Geometry: final body of the model. Coordinates: model frame, mm. Face numbers are marked on the shaded views. Coordinates: 2 decimals unless noted, no trailing zeros. Loops run counter-clockwise (first coordinate to the right, second up) from the corner with the lowest first, then second, coordinate; pieces in that order, holes last. Notation, with made-up numbers: (7.25, -11) - (53.25, -11) arc R15 cw to (53.25, 5) - close; hole circle Ø4 at (41, 60). An arc over 180 degrees is marked (long way). Put each result on its own line as item: value. Start each with the question number.
1) Material intervals for line 1 along Z through (x, y) = (0, 3.75); line 2 along Z through (x, y) = (2.5, 10.25), sorted ascending. Write a range as from..to.
2) Section A-A on z = 0. Output: boundary loops of the cut face in (x, y), and give its area (3 significant figures).
3) Section D-D on y = 13.25. Output: boundary loops of the cut face in (x, z), and give its area (3 significant figures).
4) Contact query for flat-ended pins moving along their axis: pin 1 Ø1.5 at (x, y) = (1, 3) entering from +Z; pin 2 Ø4 at (y, z) = (3.5, 0.5) entering from +X; pin 3 Ø3 at (y, z) = (11, 1) entering from -X. Output: stop coordinate, or through.
5) Draft query along X for the marked faces 1, 2, 3 and 4. Return one class per face: +X half, -X half, draft (parallel to the pull), parting line (faces both ways), or undercut.
6) Section B-B on x = 0.75. Output: boundary loops of the cut face in (y, z).
7) Section C-C on x = 3.25. Output: boundary loops of the cut face in (y, z), and give its area (3 significant figures).
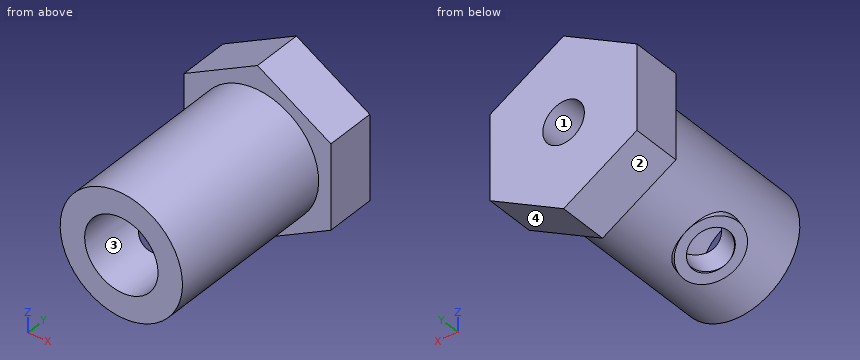
```python
from build123d import *

# Parameters (mm, degrees)
SKETCH1_R                 = 5
SKETCH1_R_2               = 3
BOSS_EXTRUDE1_DEPTH       = 14
BOSS_EXTRUDE2_DEPTH       = 4
M3_CLEARANCE_HOLE1_D      = 3.4
M3_CLEARANCE_HOLE2_REACH  = 25.495
M3_CLEARANCE_HOLE2_BORE_R = 1.7
BOSS_EXTRUDE3_REACH       = 25.495
BOSS_EXTRUDE3_END_RADIUS  = 5
SKETCH11_R                = 2.549362178
SKETCH11_R_2              = 1.7
SKETCH14_R                = 2.549362178
CUT_EXTRUDE2_DEPTH        = 1


with BuildPart() as part:
    # Sketch1 → Boss-Extrude1 (new body)
    with BuildSketch(Plane(origin=(0, 0, 0), x_dir=(1, 0, 0), z_dir=(0, 1, 0))):
        with Locations(Location((0, 0, 0), (0, 0, 270))):
            Circle(SKETCH1_R)
        with Locations(Location((0, 0, 0), (0, 0, 270))):
            Circle(SKETCH1_R_2, mode=Mode.SUBTRACT)
    extrude(amount=BOSS_EXTRUDE1_DEPTH)

    # Sketch2 → Boss-Extrude2 (add)
    with BuildSketch(Plane(origin=(0, 14, 0), x_dir=(1, 0, 0), z_dir=(0, 1, 0))):
        Polygon((0, 6.92820323), (-6, 3.464101615), (-6, -3.464101615), (0, -6.92820323), (6, -3.464101615), (6, 3.464101615), align=None)
    extrude(amount=BOSS_EXTRUDE2_DEPTH)

    # M3 Clearance Hole1 (through all)
    with Locations(Plane(origin=(0, 18, 0), x_dir=(1, 0, 0), z_dir=(0, 1, 0))):
        with Locations((0, 0)):
            Hole(M3_CLEARANCE_HOLE1_D / 2)

    # M3 Clearance Hole2 bore → M3 Clearance Hole2 (cut, up to next)
    with BuildSketch(Plane(origin=(-3, 0, -5.196152423), x_dir=(-0.8660254037844386, 0, 0.5000000000000003), z_dir=(-0.5000000000000002, 0, -0.8660254037844385)), mode=Mode.PRIVATE) as m3_clearance_hole2_sk1:
        with Locations((0, 6)):
            Circle(M3_CLEARANCE_HOLE2_BORE_R)
    m3_clearance_hole2_tool1 = extrude(m3_clearance_hole2_sk1.sketch, amount=-M3_CLEARANCE_HOLE2_REACH, mode=Mode.PRIVATE) & part.part
    add(m3_clearance_hole2_tool1.solids().sort_by_distance((-3, 6, -5.196152))[0], mode=Mode.SUBTRACT)

    # Boss-Extrude3: up to this cylinder (the profile starts outside it)
    boss_extrude3_end = Plane(origin=(0, 6, 0), z_dir=(0, -1, 0)) * Cylinder(BOSS_EXTRUDE3_END_RADIUS, 61.99, mode=Mode.PRIVATE)
    # Sketch11 → Boss-Extrude3 (add, up to the surface)
    with BuildSketch(Plane(origin=(-3, 0, -5.196152423), x_dir=(-0.8660254037844386, 0, 0.5000000000000003), z_dir=(-0.5000000000000002, 0, -0.8660254037844385)), mode=Mode.PRIVATE) as boss_extrude3_sk1:
        with Locations((0, 6)):
            Circle(SKETCH11_R)
        with Locations((0, 6)):
            Circle(SKETCH11_R_2, mode=Mode.SUBTRACT)
    boss_extrude3_tool1 = extrude(boss_extrude3_sk1.sketch, amount=-BOSS_EXTRUDE3_REACH, mode=Mode.PRIVATE) - boss_extrude3_end
    add(boss_extrude3_tool1.solids().sort_by_distance((-0.854634, 6, -6.43478))[0])

    # Sketch14 → Cut-Extrude2 (cut)
    with BuildSketch(Plane(origin=(-3, 0, -5.196152423), x_dir=(-0.8660254037844384, 0, 0.5000000000000004), z_dir=(-0.5000000000000004, 0, -0.8660254037844384))):
        with Locations((0, 6)):
            Circle(SKETCH14_R)
    extrude(amount=-CUT_EXTRUDE2_DEPTH, mode=Mode.SUBTRACT)


solid = part.part
```
Answer block:
1. line 1: z = -5..-3, 3..5
1. line 2: z = -4.33..-1.66, 1.66..4.33
2. outline: (-6, 14) - (-5, 14) - (-5, 0) - (-3, 0) - (-3, 14) - (-1.7, 14) - (-1.7, 18) - (-6, 18) - close; (1.7, 14) - (3, 14) - (3, 0) - (5, 0) - (5, 14) - (6, 14) - (6, 18) - (1.7, 18) - close
2. area: 90.4 mm²
3. outline: circle Ø10 at (0, 0); hole circle Ø6 at (0, 0)
3. area: 50.3 mm²
4. pin 1: stops at z = 4.99
4. pin 2: stops at x = 5
4. pin 3: stops at x = -5
5. face 1: undercut
5. face 2: -X half
5. face 3: undercut
5. face 4: +X half
6. outline: (0, -4.94) - (14, -4.94) - (14, -6.5) - (18, -6.5) - (18, -1.53) - (14, -1.53) - (14, -2.9) - (0, -2.9) - close; (0, 2.9) - (14, 2.9) - (14, 1.53) - (18, 1.53) - (18, 6.5) - (14, 6.5) - (14, 4.94) - (0, 4.94) - close
7. outline: (0, -3.8) - (14, -3.8) - (14, -5.05) - (18, -5.05) - (18, 5.05) - (14, 5.05) - (14, 3.8) - (0, 3.8) - close
7. area: 147 mm²
